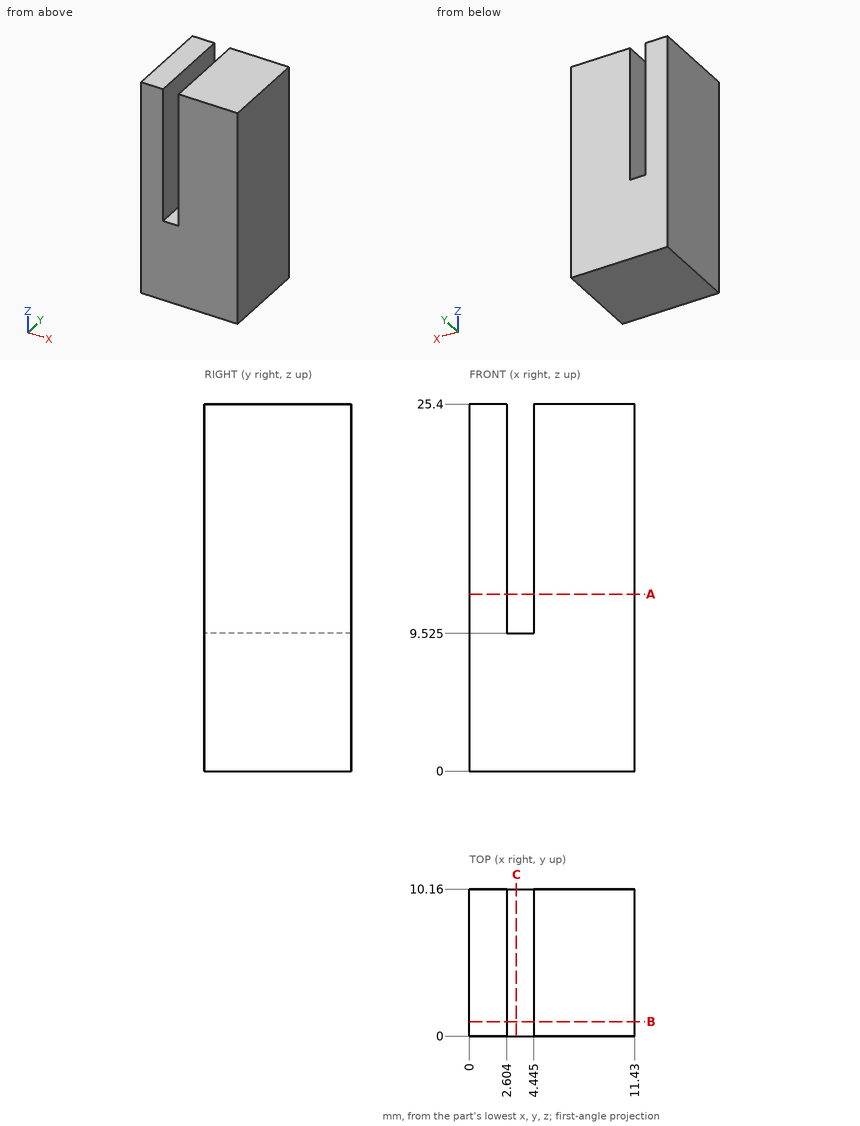
Geometry check sheet. Reference: drawing and pictorial views, mm from the part's lowest x, y, z. Round coordinates to 2 decimals unless told otherwise and drop trailing zeros. Loops run counter-clockwise (first coordinate to the right, second up) from the corner with the lowest first, then second, coordinate; pieces in that order, holes last.
1. Sectioned sample at B-B on y = 1. Record the boundary of the cut face in (x, z) (1 decimal).
2. Sectioned sample at C-C on x = 3.25. Record the boundary of the cut face in (y, z) (1 decimal).
3. Sectioned sample at A-A on z = 12.25. Record the boundary of the cut face in (x, y) (1 decimal).
4. Scan lines: probe 1 along X at (y, z) = (4, 19) (1 decimal); probe 2 along Z at (x, y) = (2.75, 2.75) (1 decimal). Record each from-to range of solid material in increasing order.
Recorded:
1. outline: (0, 0) - (11.4, 0) - (11.4, 25.4) - (4.4, 25.4) - (4.4, 9.5) - (2.6, 9.5) - (2.6, 25.4) - (0, 25.4) - close
2. outline: (0, 0) - (10.2, 0) - (10.2, 9.5) - (0, 9.5) - close
3. outline: (0, 0) - (2.6, 0) - (2.6, 10.2) - (0, 10.2) - close; (4.4, 0) - (11.4, 0) - (11.4, 10.2) - (4.4, 10.2) - close
4. probe 1: x = 0 to 2.6, 4.4 to 11.4
4. probe 2: z = 0 to 9.5
